Design review of the part built by this model. Coordinates are the model's own, in mm. Face numbers are marked on the shaded views. A direction names the side the tool comes from. Coordinates: 2 decimals unless noted, no trailing zeros. Loops run counter-clockwise (first coordinate to the right, second up) from the corner with the lowest first, then second, coordinate; pieces in that order, holes last. Notation, with made-up numbers: (71.25, 21) -> (80.25, 21) arc R32 ccw to (80.25, 56) -> close; hole circle Ø1 at (34.5, -23). An arc over 180 degrees is marked (long way). One line per item, written item: value. Start each with the question number.
1. For probe 1 along X at (y, z) = (18.5, 47); probe 2 along X at (y, z) = (5, 34.5); probe 3 along Z at (x, y) = (-14, 4), list the stretches that pass through material, from the lowest coordinate up.
2. Insertion check: pin 1 (17 mm diameter, centred on x = 9.5, y = 21.5, fed in from -Z); pin 2 (2 mm diameter, centred on x = 66, z = -5.5, fed in from +Y); pin 3 (0.7 mm diameter, centred on x = -66, y = 4, fed in from -Z). Each pin has a flat end and moves straight along its axis. Give the tip position at first contact, or say it passes through.
3. Add section A-A on z = 62.5. Write out the cut boundary in (x, y).
4. Machinability: for the marked faces 4 and 5, which of the approach directions +Z, -Z, +X, -X, +Y, -Y give a long, thin tool a straight path to every point of the face, cutting with its end or side? Answer none if there is none.
5. Add section C-C on x = 18.5. Write out the cut boundary in (y, z).
6. Draft analysis for pull direction X (two halves, no side actions). For the marked faces 1, 2 and 3, state which applies: pulls with the +X half, pulls with the -X half, needs draft (parallel to the pull), parting line crosses it, or undercut.
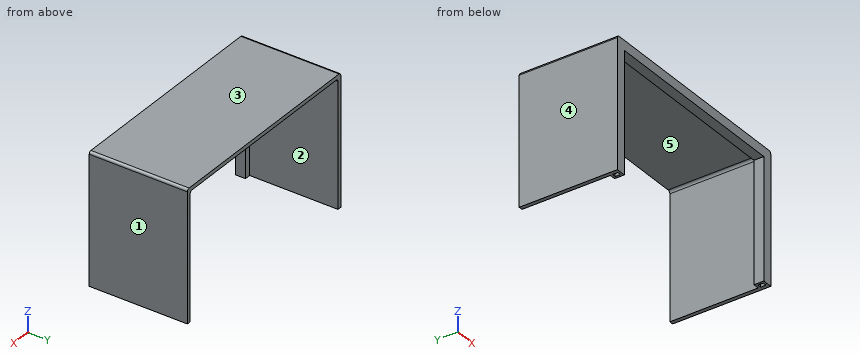
```python
from build123d import *

# Parameters (mm, degrees)
SKETCH1_W           = 139.7
SKETCH1_H           = 154.20848
BOSS_EXTRUDE1_DEPTH = 6.35
SKETCH2_W           = 127
SKETCH2_H           = 141.50848
CUT_EXTRUDE1_DEPTH  = 6.35
SKETCH3_W           = 139.7
SKETCH3_H           = 154.20848
SKETCH3_W_2         = 134.62
SKETCH3_H_2         = 149.12848
BOSS_EXTRUDE2_DEPTH = 57.15
SKETCH4_W           = 139.7
SKETCH4_H           = 69.85
CUT_EXTRUDE2_DEPTH  = 64.5
SKETCH5_W           = 2.4765
SKETCH5_H           = 3.429
CUT_EXTRUDE3_DEPTH  = 3.81
FILLET1_R           = 1.5875


with BuildPart() as part:
    # Sketch1 → Boss-Extrude1 (new body)
    with BuildSketch(Plane(origin=(0, 0, 0), x_dir=(1, 0, 0), z_dir=(0, 1, 0))):
        Rectangle(SKETCH1_W, SKETCH1_H)
    extrude(amount=BOSS_EXTRUDE1_DEPTH)

    # Sketch2 → Cut-Extrude1 (cut)
    with BuildSketch(Plane(origin=(0, 6.35, 0), x_dir=(1, 0, 0), z_dir=(0, 1, 0))):
        Rectangle(SKETCH2_W, SKETCH2_H)
    extrude(amount=-CUT_EXTRUDE1_DEPTH, mode=Mode.SUBTRACT)

    # Sketch3 → Boss-Extrude2 (add)
    with BuildSketch(Plane(origin=(0, 6.35, 0), x_dir=(1, 0, 0), z_dir=(0, 1, 0))):
        Rectangle(SKETCH3_W, SKETCH3_H)
        Rectangle(SKETCH3_W_2, SKETCH3_H_2, mode=Mode.SUBTRACT)
    extrude(amount=BOSS_EXTRUDE2_DEPTH)

    # Sketch4 → Cut-Extrude2 (cut, through all)
    with BuildSketch(Plane(origin=(0, 63.5, 0), x_dir=(1, 0, 0), z_dir=(0, 1, 0))):
        with Locations((0, 42.17924)):
            Rectangle(SKETCH4_W, SKETCH4_H)
    extrude(amount=-CUT_EXTRUDE2_DEPTH, mode=Mode.SUBTRACT)

    # Sketch5 → Cut-Extrude3 (cut)
    with BuildSketch(Plane(origin=(0, 0, -7.25424), x_dir=(-1, 0, 0), z_dir=(0, 0, -1))):
        with Locations((66.19875, 3.175)):
            Rectangle(SKETCH5_W, SKETCH5_H)
        with Locations((-66.19875, 3.175)):
            Rectangle(SKETCH5_W, SKETCH5_H)
    extrude(amount=-CUT_EXTRUDE3_DEPTH, mode=Mode.SUBTRACT)

    # Fillet1
    fillet1_edges = [part.edges().sort_by_distance(p)[0] for p in [
        (-67.31, 34.925, 74.56424),
        (67.31, 34.925, 74.56424),
        (69.85, 31.75, 77.10424),
        (-69.85, 31.75, 77.10424),
    ]]
    fillet(fillet1_edges, radius=FILLET1_R)


solid = part.part
```
Worked answers:
1. probe 1: x = -69.85 to -67.31, 67.31 to 69.85
1. probe 2: x = -69.85 to -63.5, 63.5 to 69.85
1. probe 3: z = 70.75 to 77.1
2. pin 1: stops at z = 74.56
2. pin 2: stops at y = 6.35
2. pin 3: stops at z = -3.44
3. outline: (-69.85, 0) -> (-63.5, 0) -> (-63.5, 6.35) -> (-67.31, 6.35) -> (-67.31, 63.5) -> (-69.85, 63.5) -> close; (63.5, 0) -> (69.85, 0) -> (69.85, 63.5) -> (67.31, 63.5) -> (67.31, 6.35) -> (63.5, 6.35) -> close
4. face 4: +Z, -Z, -X, +Y, -Y
4. face 5: -Z, +Y
5. outline: (0, 70.75) -> (6.35, 70.75) -> (6.35, 74.56) -> (63.5, 74.56) -> (63.5, 77.1) -> (0, 77.1) -> close
6. face 1: pulls with the +X half
6. face 2: undercut
6. face 3: needs draft
